Autodesk Inventor part; units mm, degrees
ref_plane "YZ Plane" through (0, 0, 0) normal (1, 0, 0) x (0, 1, 0)
ref_plane "XZ Plane" through (0, 0, 0) normal (0, 1, 0) x (-1, 0, 0)
ref_plane "XY Plane" through (0, 0, 0) normal (0, 0, 1) x (1, 0, 0)
sketch "Sketch1" plane through (0, 0, 0) normal (0, 0, 1) x (1, 0, 0)
  line L0 (20, 100) -> (0, 100)
  line L1 (0, 100) -> (0, 45.15)
  line L2 (0, 45.15) -> (0, 0) construction
  line L3 (0, 0) -> (20, 0) construction
  line L4 (20, 100) -> (20, 45.15)
  line L5 (20, 45.15) -> (0, 45.15)
  line L6 (20, 45.15) -> (20, 0) construction
  dimension "d0" = 200
  dimension "d1" = 20
  dimension "d5" = 90.3
revolve "Revolution1" add sketch "Sketch1" angle 360 about axis through (0, 0, 0) along (1, 0, 0)
sketch "Sketch2" plane through (0, 0, 0) normal (-1, 0, 0) x (0, 0, 1)
  circle A0 centre (0, 0) radius 45.15
  line L0 (0, 80) -> (0, 0) construction
  circle A1 centre (0, 0) radius 100
  circle A2 centre (0, 0) radius 80 construction
  line L1 (0, 0) -> (30.6147, 73.9104) construction
  circle A3 centre (30.6147, 73.9104) radius 9
  dimension "d6" = 18
  dimension "d7" = 80
  dimension "d8" = 22.5
extrude "Extrusion1" cut sketch "Sketch2" against normal through all contours A3
pattern_circular "Circular Pattern1" count 8 over 360 about axis through (10, 0, 0) along (1, 0, 0) of "Extrusion1"
equation "\"d6\" = dd2"
equation "\"d7\" = 0.5 * k"
equation "\"d0\" = D"
equation "\"d1\" = b"
equation "\"d5\" = dd5"
equation "\"b\" = 20"
equation "\"D\" = 200"
equation "\"dd2\" = 18"
equation "\"dd5\" = 90.3"
equation "\"Size_Designation\" = 1.2345"
properties part number "DIN 2576 Slip-On Flange for Welding Series 1 (ISO) - PN 10 80 x 88.9" material "Steel"
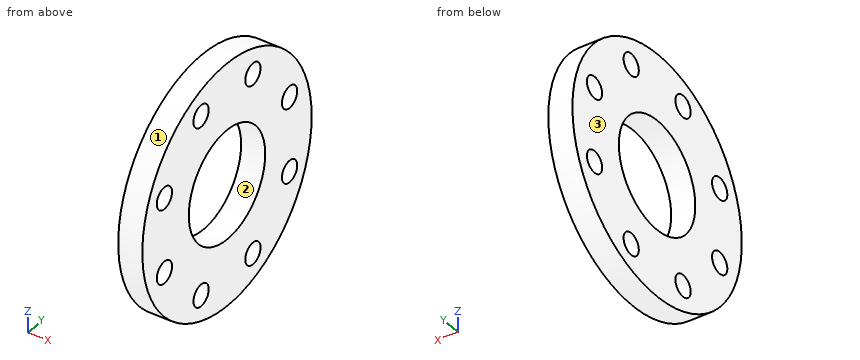
Check sheet for the modelled part. Datum: model origin and axes. Units: mm. Face numbers are marked on the shaded views. Round coordinates to 2 decimals unless told otherwise and drop trailing zeros. Order: outer loops, then holes, each group sorted by start corner. A loop starts at its lowest first (then second) coordinate and runs counter-clockwise, first axis right, second up. Notation, with made-up numbers: M 58,35 L 78,35 A10 ccw 78,53 Z; hole C 52,30.5 d5. An arc over 180 degrees is marked long. Answer in a Markdown table with one row per item.
(1) Section check C-C on x = 11.25. Give the number of separate pieces and of enclosed holes in the cut face, plus the area to 3 significant figures.
Findings:
| item | result |
|---|---|
| separate pieces | 1 |
| enclosed holes | 9 |
| area | 23,000 mm^2 |
(2) Section check D-D on y = 58. Record the boundary of the cut face in (x, z), plus the area to 3 significant figures.
Findings:
| item | result |
|---|---|
| outline | M 0,-81.46 L 20,-81.46 L 20,81.46 L 0,81.46 Z |
| area | 3,260 mm^2 |
(3) Material ranges on line 1 along Z through (x, y) = (7.75, -31.5); line 2 along Y through (x, z) = (3, -30); line 3 along Z through (x, y) = (13.75, 76.5), recorded low to high. Write a range as from..to.
Findings:
| item | result |
|---|---|
| line 1 | z = -94.91..-82.87, -64.95..-32.35, 32.35..64.95, 82.87..94.91 |
| line 2 | y = -95.39..-82.89, -64.93..-33.74, 33.74..64.93, 82.89..95.39 |
| line 3 | z = -64.4..-39.23, -22..22, 39.23..64.4 |
(4) Draft check along Z on the marked faces 1, 2 and 3. Enter one of: +Z half, -Z half, draft (parallel to the pull), parting line (faces both ways), or undercut.
Findings:
| item | result |
|---|---|
| face 1 | parting line |
| face 2 | undercut |
| face 3 | draft |
(5) Gauge pin test, flat ends, axial feed: pin 1 (4 mm diameter, centred on x = 16.5, z = 23.5, fed in from -Y); pin 2 (5 mm diameter, centred on x = 2, z = -78, fed in from -Y); pin 3 (11 mm diameter, centred on y = -30.61, z = 73.91, fed in from +X); pin 4 (8 mm diameter, centred on x = 8, z = 17.5, fed in from +Y). Record the tip position at first contact, or that the pin passes through.
Findings:
| item | result |
|---|---|
| pin 1 | stops at y = -97.66 |
| pin 2 | stops at y = -65.57 |
| pin 3 | passes through |
| pin 4 | stops at y = 99.08 |
(6) Section check A-A on z = 0. Record the boundary of the cut face in (x, y), plus the area to 3 significant figures.
Findings:
| item | result |
|---|---|
| outline | M 0,-100 L 20,-100 L 20,-45.15 L 0,-45.15 Z; M 0,45.15 L 20,45.15 L 20,100 L 0,100 Z |
| area | 2,190 mm^2 |
